```python
from build123d import *

# Parameters (mm, degrees)
SKETCH3_W           = 7
SKETCH3_H           = 7
BOSS_EXTRUDE2_DEPTH = 4
SKETCH4_R           = 2
BOSS_EXTRUDE3_DEPTH = 15


with BuildPart() as part:
    # Sketch3 → Boss-Extrude2 (new body)
    with BuildSketch(Plane(origin=(0, 0, 0), x_dir=(0, 0, -1), z_dir=(1, 0, 0))):
        Rectangle(SKETCH3_W, SKETCH3_H)
    extrude(amount=BOSS_EXTRUDE2_DEPTH)

    # Sketch4 → Boss-Extrude3 (add)
    with BuildSketch(Plane(origin=(4, 0, 0), x_dir=(0, 0, -1), z_dir=(1, 0, 0))):
        Circle(SKETCH4_R)
    extrude(amount=BOSS_EXTRUDE3_DEPTH)


solid = part.part
```
Here's how the part is built. I have some questions about the finished solid (model axes, mm). A direction names the side the tool comes from. Round coordinates to 2 decimals unless told otherwise and drop trailing zeros. Order: outer loops, then holes, each group sorted by start corner. A loop starts at its lowest first (then second) coordinate and runs counter-clockwise, first axis right, second up. Notation, with made-up numbers: M 57,-2 L 104,-2 A28 cw 104,29 Z; hole C 41.25,82.5 d8. An arc over 180 degrees is marked long. Answer as CSV lines item,"result".
Item 1: Imagine slicing it at A-A on z = 0. List the corners of the cut face in (x, y) for me.
From the geometry:
outline,"M 0,-3.5 L 4,-3.5 L 4,-2 L 19,-2 L 19,2 L 4,2 L 4,3.5 L 0,3.5 Z"
Item 2: Please list where these lines run through material, in increasing order: L1, parallel to X at y = -1, z = 2.5; L2, parallel to Z at x = 12.5, y = -0.25; L3, parallel to Z at x = 10.75, y = -1. Write a range as [from, to].
From the geometry:
L1,"[0, 4]"
L2,"[-1.98, 1.98]"
L3,"[-1.73, 1.73]"
Item 3: For pin 1 (1 mm diameter, centred on x = 5.5, z = -0.5, fed in from +Y); pin 2 (1 mm diameter, centred on x = 6, y = 0.5, fed in from +Z), each with a flat end and sliding along its axis, tell me the tip position at first contact or that it passes through.
From the geometry:
pin 1,"y = 2"
pin 2,"z = 2"
Item 4: Which directions (+Z, -Z, +X, -X, +Y, -Y) give clear straight access to the entire face, cutting with the end or side of a thin tool? Please do faces 1 (the flat face through (0, 0, 0)), 2 (the cylindrical face through (11, -2, 0)).
From the geometry:
face 1,"+Z, -Z, -X, +Y, -Y"
face 2,"+X"
Item 5: Imagine slicing it at D-D on y = -2.25. List the corners of the cut face in (x, z) for me, and give its area (3 significant figures).
From the geometry:
outline,"M 0,-3.5 L 4,-3.5 L 4,3.5 L 0,3.5 Z"
area,"28.0 mm2"
Item 6: Imagine slicing it at C-C on x = 11.5. List the corners of the cut face in (y, z) for me, and give its area (3 significant figures).
From the geometry:
outline,"C 0,0 d4"
area,"12.6 mm2"
